Autodesk Inventor part; units mm, degrees
ref_plane "YZ Plane" through (0, 0, 0) normal (1, 0, 0) x (0, 1, 0)
ref_plane "XZ Plane" through (0, 0, 0) normal (0, 1, 0) x (-1, 0, 0)
ref_plane "XY Plane" through (0, 0, 0) normal (0, 0, 1) x (1, 0, 0)
sketch "Náčrt1" plane through (0, 0, 0) normal (0, 0, 1) x (1, 0, 0)
  line L0 (47.8317, -5) -> (50.8317, -5)
  line L1 (50.8317, -5) -> (50.8317, 5)
  line L2 (50.8317, 5) -> (47.8317, 5)
  line L3 (47.8317, 5) -> (47.8317, -5)
  line L4 (47.8317, -5) -> (50.8317, 5) construction
  line L5 (50.8317, -5) -> (47.8317, 5) construction
  circle A0 centre (-58.7223, 35.7005) radius 1.45
  circle A1 centre (-58.7223, -35.5995) radius 1.45
  point P0 (0, 0)
  point P1 (50.8317, 0)
  point P2 (-60.1683, 0.0505)
  dimension "d7" = 10
  dimension "d8" = 5
  dimension "d13" = 2.9
  dimension "d14" = 74.2
extrude "Vysunutí1" add sketch "Náčrt1" along normal blind 17
sketch "Náčrt2" plane through (-58.7223, 35.7005, 17) normal (0, 0, 1) x (1, 0, 0)
  circle A0 centre (0, 0) radius 1.45
  line L0 (109.5541, -40.7005) -> (109.5541, -30.7005)
  arc A1 (0.9632, 1.0839) -> (109.5541, -30.7005) centre (125.5077, 225.1962) ccw
  circle A2 centre (0, -71.3) radius 1.45
  line L1 (-1.45, 0) -> (-1.45, -71.3)
  arc A3 (109.5541, -40.7005) -> (0.9632, -72.3839) centre (125.3027, -296.61) ccw
  arc A4 (1.55, -3.0822) -> (1.9226, -2.8646) centre (0, 0) ccw
  line L2 (106.5541, -33.504) -> (106.5541, -37.8971)
  arc A5 (106.5541, -37.8971) -> (1.8423, -68.4842) centre (125.3027, -296.61) ccw
  arc A6 (1.8423, -68.4842) -> (1.55, -68.3189) centre (0, -71.4011) ccw
  line L3 (106.5541, -37.8971) -> (106.5541, -33.504)
  line L4 (1.55, -3.0822) -> (1.55, -68.3189)
  arc A7 (1.9226, -2.8646) -> (106.5541, -33.504) centre (125.5077, 225.1962) ccw
  line L5 (109.5541, -30.7005) -> (109.5541, -40.7005)
  arc A8 (0.4127, -72.69) -> (0.9632, -72.3839) centre (0, -71.3) ccw
  arc A9 (0.9632, 1.0839) -> (-1.45, 0) centre (0, 0) ccw
  arc A10 (0.9632, 1.0839) -> (-1.45, 0) centre (0, 0) ccw
  arc A11 (-1.45, -71.3) -> (0.9632, -72.3839) centre (0, -71.3) ccw
  point P0 (58.7223, -35.7005)
  point P1 (3.4391, -0.2742)
  point P2 (-1.45, -3.1305)
  point P3 (3.4391, -71.1268)
  point P4 (-1.45, -68.2706)
  point P5 (109.5541, -35.7005)
  point P6 (106.5541, -35.7005)
  dimension "d20" = 2
  dimension "d23" = 3
extrude "Vysunutí2" add sketch "Náčrt2" along normal blind 5
properties part number "drzak_baterie"
Source: CAD feature listing. Evaluate the final solid. Frame: model axes, mm. A direction names the side the tool comes from. Coordinates: 2 decimals unless noted, no trailing zeros. Write each loop counter-clockwise with the first axis right and the second up, starting at its lowest first coordinate (ties: lowest second). Pieces come first, ordered by that corner, then holes. Notation, with made-up numbers: (29.25, 61) -> (40.25, 61) arc R16 ccw to (40.25, 83) -> close; hole circle Ø1 at (0, 25). An arc over 180 degrees is marked (long way). Return JSON: item names as keys, results as strings. Group by question number.
1) Contact query for flat-ended pins moving along their axis: P1, Ø12, axis at y = 21, z = 9, coming from the +X side; P2, Ø0.9, axis at x = 49.5, z = 4.5, coming from the -Y side; P3, Ø12, axis at y = -3.5, z = 6.5, coming from the -X side; P4, Ø6, axis at x = -42, y = 22.5, coming from the -Z side. Output: stop coordinate, or through.
2) Ray query, line 1 along Y through (x, z) = (35, 21); line 2 along Z through (x, y) = (-53.5, 33.5); line 3 along X through (y, z) = (-30, 20.25). Return the intervals inside material, ascending.
3) Section query B-B, the plane z = 13. Return loops of the section in (x, y), plus the area to 3 significant figures.
4) Section query C-C, the plane x = -17. Return loops of the section in (y, z).
5) Set-up query: faces 4 (the face through (47.832, 0, 8)), 5 (the face through (-57.172, 0, 19)), 6 (the face through (-59.79, -36.58, 10.85)), 7 (the face through (49, 5, 8)). Return all of +Z, -Z, +X, -X, +Y, -Y with unobstructed straight access to the full face (end or side cutting, diameter ignored); none if empty.
6) Mould query, pull axis Y, two halves, no side actions, for faces 1 (the face through (50.832, 0, 8)), 2 (the face through (-4.472, 14.604, 19.465)), 3 (the face through (-6.89, -12.14, 19.46)). Classes: +Y half, -Y half, draft (parallel to the pull), parting line (faces both ways), or undercut.
7) Section query D-D, the plane y = 14. Return loops of the section in (x, z), plus the area to 3 significant figures.
From the geometry:
{
 "1": {"P1": "through", "P2": "y = -5", "P3": "x = 47.83", "P4": "z = 17"},
 "2": {"line 1": "-6.47 to -3.45, 3.46 to 6.48", "line 2": "17 to 22", "line 3": "-60.17 to -57.17, -51.59 to -44.86"},
 "3": {"outline": "circle Ø2.9 at (-58.72, -35.6); circle Ø2.9 at (-58.72, 35.7); (47.83, -5) -> (50.83, -5) -> (50.83, 5) -> (47.83, 5) -> close", "area": "43.2 mm²"},
 "4": {"outline": "(-18.52, 17) -> (-15.35, 17) -> (-15.35, 22) -> (-18.52, 22) -> close; (15.41, 17) -> (18.58, 17) -> (18.58, 22) -> (15.41, 22) -> close"},
 "5": {"face 4": "-Z, -X, +Y, -Y", "face 5": "+Z, -Z", "face 6": "-Z", "face 7": "-Z, +X, -X, +Y"},
 "6": {"face 1": "draft", "face 2": "+Y half", "face 3": "undercut"},
 "7": {"outline": "(-60.17, 17) -> (-57.17, 17) -> (-57.17, 22) -> (-60.17, 22) -> close; (-12.76, 17) -> (-2.35, 17) -> (-2.35, 22) -> (-12.76, 22) -> close", "area": "67.0 mm²"}
}
